Design review of the part built by this model. Coordinates are the model's own, in mm. Face numbers are marked on the shaded views. A direction names the side the tool comes from. Coordinates: 2 decimals unless noted, no trailing zeros. Loops run counter-clockwise (first coordinate to the right, second up) from the corner with the lowest first, then second, coordinate; pieces in that order, holes last. Notation, with made-up numbers: M 29.25,46 L 72.25,46 A21 cw 72.25,62 Z; hole C -9.5,72 d9. An arc over 180 degrees is marked long. Answer as a JSON object with one key per item and string values. Group by question number.
1. Consider section A-A (z = 0). State the section outline as (x, y) points.
2. Consider section C-C (x = 70). State the section outline as (y, z) points, then the cut area to 3 significant figures.
3. Consider section D-D (z = 15.5). State the section outline as (x, y) points.
4. To check wall thickness, follow probe 1 along X at (y, z) = (1.7, 0); probe 2 along X at (y, z) = (0.2, 18); probe 3 along Y at (x, z) = (70, -3). State the ranges of each line that lie inside material, in increasing order.
5. Consider section B-B (y = 2.2). State the section outline as (x, z) points.
6. Machinability: for the marked faces 1 and 2, which of the approach directions +Z, -Z, +X, -X, +Y, -Y give a long, thin tool a straight path to every point of the face, cutting with its end or side? Answer none if there is none.
7. Insertion check: pin 1 (1.2 mm diameter, centred on x = 69, y = 1, fed in from -Z); pin 2 (2 mm diameter, centred on x = 71.5, z = -10.5, fed in from +Y); pin 3 (1.6 mm diameter, centred on x = 70.5, y = 1, fed in from +Z). Each pin has a flat end and moves straight along its axis. Give the tip position at first contact, or say it passes through.
from build123d import *

# Parameters (mm, degrees)
CROQUIS1_R                 = 11
CROQUIS1_R_2               = 2
CROQUIS1_W                 = 30
CROQUIS1_H                 = 3
SALIENTE_EXTRUIR1_DEPTH    = 3
CROQUIS2_R                 = 13
CROQUIS2_R_2               = 11
SALIENTE_EXTRUIR2_DEPTH    = 4
CROQUIS3_R                 = 13
CROQUIS3_R_2               = 9
SALIENTE_EXTRUIR3_DEPTH    = 2
CHAFL_N1_SIZE              = 2
CHAFL_N2_SIZE              = 10
CROQUIS6_W                 = 10
CROQUIS6_H                 = 20
CROQUIS6_R                 = 2.5
CORTAR_EXTRUIR2_DEPTH      = 1.5
CORTAR_EXTRUIR3_DEPTH      = 10
CORTAR_EXTRUIR3_DEPTH_BACK = 10
CROQUIS7_OUTSIDE_W         = 171.176
CROQUIS7_OUTSIDE_H         = 71.176
CROQUIS7_OUTSIDE_W_2       = 13.478659513
CROQUIS7_OUTSIDE_H_2       = 41.596343219


with BuildPart() as part:
    # Croquis1 → Saliente-Extruir1 (new body)
    with BuildSketch(Plane(origin=(0, 0, 0), x_dir=(1, 0, 0), z_dir=(0, 1, 0))):
        Polygon((-65, -20), (65, -20), (65, -10), (75, -10), (75, 10), (65, 10), (65, 20), (-65, 20), align=None)
        with Locations(Location((-50.129942902, 0, 0), (0, 0, 270))):
            Circle(CROQUIS1_R, mode=Mode.SUBTRACT)
        with Locations(Location((-28.595127909, 0, 0), (0, 0, 270))):
            Circle(CROQUIS1_R_2, mode=Mode.SUBTRACT)
        with Locations(Location((-13.595127909, 0, 0), (0, 0, 270))):
            Circle(CROQUIS1_R_2, mode=Mode.SUBTRACT)
        with Locations(Location((50, 0, 0), (0, 0, 270))):
            Circle(CROQUIS1_R_2, mode=Mode.SUBTRACT)
        with Locations((25, 11)):
            Rectangle(CROQUIS1_W, CROQUIS1_H, mode=Mode.SUBTRACT)
        with Locations((25, -11)):
            Rectangle(CROQUIS1_W, CROQUIS1_H, mode=Mode.SUBTRACT)
    extrude(amount=SALIENTE_EXTRUIR1_DEPTH)

    # Croquis2 → Saliente-Extruir2 (add)
    with BuildSketch(Plane(origin=(0, 3, 0), x_dir=(1, 0, 0), z_dir=(0, 1, 0))):
        with Locations(Location((-50.129942902, 0, 0), (0, 0, 90))):
            Circle(CROQUIS2_R)
        with Locations(Location((-50.129942902, 0, 0), (0, 0, 270))):
            Circle(CROQUIS2_R_2, mode=Mode.SUBTRACT)
    extrude(amount=SALIENTE_EXTRUIR2_DEPTH)

    # Croquis3 → Saliente-Extruir3 (add)
    with BuildSketch(Plane(origin=(0, 7, 0), x_dir=(1, 0, 0), z_dir=(0, 1, 0))):
        with Locations(Location((-50.129942902, 0, 0), (0, 0, 90))):
            Circle(CROQUIS3_R)
        with Locations(Location((-50.129942902, 0, 0), (0, 0, 270))):
            Circle(CROQUIS3_R_2, mode=Mode.SUBTRACT)
    extrude(amount=SALIENTE_EXTRUIR3_DEPTH)

    # Chafl_n1
    chafl_n1_edges = [part.edges().sort_by_distance(p)[0] for p in [
        (-50.129942902, 9, 13),
    ]]
    chamfer(chafl_n1_edges, length=CHAFL_N1_SIZE)

    # Chafl_n2
    chafl_n2_edges = [part.edges().sort_by_distance(p)[0] for p in [
        (-65, 1.5, 20),
        (-65, 1.5, -20),
    ]]
    chamfer(chafl_n2_edges, length=CHAFL_N2_SIZE)

    # Croquis6 → Cortar-Extruir2 (cut)
    with BuildSketch(Plane(origin=(0, 3, 0), x_dir=(1, 0, 0), z_dir=(0, 1, 0))):
        with Locations((70, 0)):
            Rectangle(CROQUIS6_W, CROQUIS6_H)
        with Locations(Location((70, 0, 0), (0, 0, 270))):
            Circle(CROQUIS6_R, mode=Mode.SUBTRACT)
    extrude(amount=-CORTAR_EXTRUIR2_DEPTH, mode=Mode.SUBTRACT)

    # Croquis7 outside → Cortar-Extruir3 (cut, two sides: drawn at the far end of the back side and taken through both)
    with BuildSketch(Plane(origin=(0, 3, 0), x_dir=(1, 0, 0), z_dir=(0, 1, 0)).offset(-CORTAR_EXTRUIR3_DEPTH_BACK)):
        with Locations((5, 0)):
            Rectangle(CROQUIS7_OUTSIDE_W, CROQUIS7_OUTSIDE_H)
        with Locations((69.759812965, -0.79817161)):
            Rectangle(CROQUIS7_OUTSIDE_W_2, CROQUIS7_OUTSIDE_H_2, mode=Mode.SUBTRACT)
    extrude(amount=CORTAR_EXTRUIR3_DEPTH + CORTAR_EXTRUIR3_DEPTH_BACK, mode=Mode.SUBTRACT)


solid = part.part
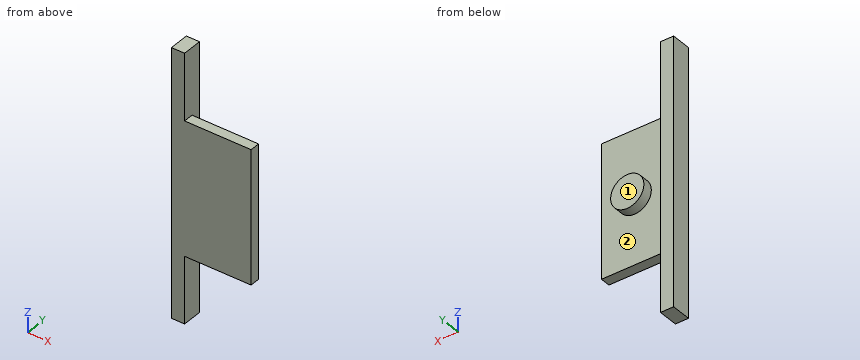
Findings below:
{
 "1": {"outline": "M 63.02,0 L 75,0 L 75,1.5 L 72.5,1.5 L 72.5,3 L 67.5,3 L 67.5,1.5 L 65,1.5 L 65,3 L 63.02,3 Z"},
 "2": {"outline": "M 0,-10 L 1.5,-10 L 1.5,-2.5 L 3,-2.5 L 3,2.5 L 1.5,2.5 L 1.5,10 L 0,10 Z", "area": "37.5 mm^2"},
 "3": {"outline": "M 63.02,0 L 65,0 L 65,3 L 63.02,3 Z"},
 "4": {"probe 1": "x = 63.02 to 65, 67.5 to 72.5", "probe 2": "x = 63.02 to 65", "probe 3": "y = 0 to 1.5"},
 "5": {"outline": "M 63.02,-20 L 65,-20 L 65,20 L 63.02,20 Z; C 70,0 d5"},
 "6": {"face 1": "+Z, -Z, +X, -X, +Y", "face 2": "+Y"},
 "7": {"pin 1": "stops at z = -10", "pin 2": "stops at y = 1.5", "pin 3": "stops at z = 10"}
}
